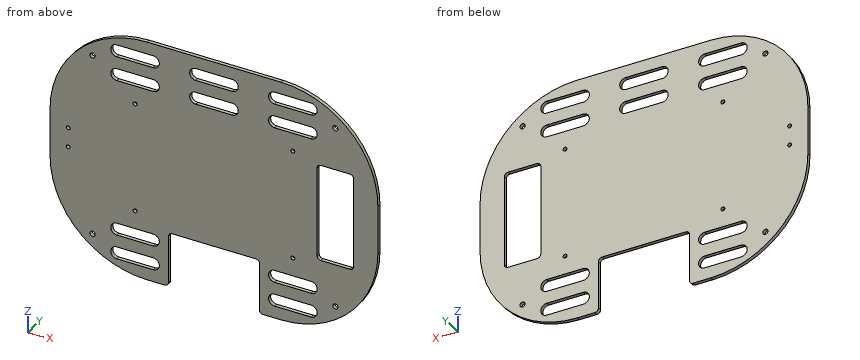
from build123d import *

# Parameters (mm, degrees)
SKETCH_1_W          = 270
SKETCH_1_H          = 200
EXTRUDE_1_DEPTH     = 3
SKETCH_2_R          = 2.15
CUT_EXTRUDE_1_DEPTH = 3
SKETCH_3_R          = 1.6
CUT_EXTRUDE_2_DEPTH = 3
SKETCH_4_W          = 75
SKETCH_4_H          = 45
CUT_EXTRUDE_3_DEPTH = 3
SKETCH_5_R          = 1.6
CUT_EXTRUDE_4_DEPTH = 3
SKETCH_6_W          = 30
SKETCH_6_H          = 80
CUT_EXTRUDE_5_DEPTH = 3
CUT_EXTRUDE_6_DEPTH = 3
FILLET_1_R          = 3


with BuildPart() as part:
    # 草图1 → 凸台-拉伸1 (new body)
    with BuildSketch(Plane(origin=(0, 0, 0), x_dir=(1, 0, 0), z_dir=(0, 1, 0))):
        Rectangle(SKETCH_1_W, SKETCH_1_H)
    extrude(amount=EXTRUDE_1_DEPTH)

    # 草图2 → 切除-拉伸1 (cut)
    with BuildSketch(Plane(origin=(0, 3, 0), x_dir=(1, 0, 0), z_dir=(0, 1, 0))):
        with Locations(Location((-100, 75, 0), (0, 0, 270))):
            Circle(SKETCH_2_R)
        with Locations(Location((100, 75, 0), (0, 0, 270))):
            Circle(SKETCH_2_R)
        with Locations(Location((100, -75, 0), (0, 0, 270))):
            Circle(SKETCH_2_R)
        with Locations(Location((-100, -75, 0), (0, 0, 270))):
            Circle(SKETCH_2_R)
    extrude(amount=-CUT_EXTRUDE_1_DEPTH, mode=Mode.SUBTRACT)

    # 草图3 → 切除-拉伸2 (cut)
    with BuildSketch(Plane(origin=(0, 3, 0), x_dir=(1, 0, 0), z_dir=(0, 1, 0))):
        with Locations(Location((-120, 8, 0), (0, 0, 270))):
            Circle(SKETCH_3_R)
        with Locations(Location((-120, -8, 0), (0, 0, 270))):
            Circle(SKETCH_3_R)
    extrude(amount=-CUT_EXTRUDE_2_DEPTH, mode=Mode.SUBTRACT)

    # 草图4 → 切除-拉伸3 (cut)
    with BuildSketch(Plane(origin=(0, 3, 0), x_dir=(1, 0, 0), z_dir=(0, 1, 0))):
        with BuildLine():
            Line((-80, -80), (-50, -80))
            ThreePointArc((-50, -80), (-45, -85), (-50, -90))
            Line((-50, -90), (-80, -90))
            ThreePointArc((-80, -90), (-85, -85), (-80, -80))
        make_face()
        with BuildLine():
            Line((-15, -80), (15, -80))
            ThreePointArc((15, -80), (20, -85), (15, -90))
            Line((15, -90), (-15, -90))
            ThreePointArc((-15, -90), (-20, -85), (-15, -80))
        make_face()
        with BuildLine():
            Line((50, -80), (80, -80))
            ThreePointArc((80, -80), (85, -85), (80, -90))
            Line((80, -90), (50, -90))
            ThreePointArc((50, -90), (45, -85), (50, -80))
        make_face()
        with BuildLine():
            Line((-15, -60), (15, -60))
            ThreePointArc((15, -60), (20, -65), (15, -70))
            Line((15, -70), (-15, -70))
            ThreePointArc((-15, -70), (-20, -65), (-15, -60))
        make_face()
        with BuildLine():
            Line((50, -60), (80, -60))
            ThreePointArc((80, -60), (85, -65), (80, -70))
            Line((80, -70), (50, -70))
            ThreePointArc((50, -70), (45, -65), (50, -60))
        make_face()
        with BuildLine():
            Line((-80, -60), (-50, -60))
            ThreePointArc((-50, -60), (-45, -65), (-50, -70))
            Line((-50, -70), (-80, -70))
            ThreePointArc((-80, -70), (-85, -65), (-80, -60))
        make_face()
        with BuildLine():
            Line((-80, 80), (-50, 80))
            ThreePointArc((-50, 80), (-45, 85), (-50, 90))
            Line((-50, 90), (-80, 90))
            ThreePointArc((-80, 90), (-85, 85), (-80, 80))
        make_face()
        with BuildLine():
            Line((50, 80), (80, 80))
            ThreePointArc((80, 80), (85, 85), (80, 90))
            Line((80, 90), (50, 90))
            ThreePointArc((50, 90), (45, 85), (50, 80))
        make_face()
        with BuildLine():
            Line((50, 60), (80, 60))
            ThreePointArc((80, 60), (85, 65), (80, 70))
            Line((80, 70), (50, 70))
            ThreePointArc((50, 70), (45, 65), (50, 60))
        make_face()
        with BuildLine():
            Line((-80, 60), (-50, 60))
            ThreePointArc((-50, 60), (-45, 65), (-50, 70))
            Line((-50, 70), (-80, 70))
            ThreePointArc((-80, 70), (-85, 65), (-80, 60))
        make_face()
        with Locations((0, 77.5)):
            Rectangle(SKETCH_4_W, SKETCH_4_H)
    extrude(amount=-CUT_EXTRUDE_3_DEPTH, mode=Mode.SUBTRACT)

    # 草图5 → 切除-拉伸4 (cut)
    with BuildSketch(Plane(origin=(0, 3, 0), x_dir=(1, 0, 0), z_dir=(0, 1, 0))):
        with Locations(Location((-65, -45, 0), (0, 0, 270))):
            Circle(SKETCH_5_R)
        with Locations(Location((-65, 45, 0), (0, 0, 270))):
            Circle(SKETCH_5_R)
        with Locations(Location((65, 45, 0), (0, 0, 270))):
            Circle(SKETCH_5_R)
        with Locations(Location((65, -45, 0), (0, 0, 270))):
            Circle(SKETCH_5_R)
    extrude(amount=-CUT_EXTRUDE_4_DEPTH, mode=Mode.SUBTRACT)

    # 草图6 → 切除-拉伸5 (cut)
    with BuildSketch(Plane(origin=(0, 3, 0), x_dir=(1, 0, 0), z_dir=(0, 1, 0))):
        with Locations((100, 0)):
            Rectangle(SKETCH_6_W, SKETCH_6_H)
    extrude(amount=-CUT_EXTRUDE_5_DEPTH, mode=Mode.SUBTRACT)

    # 草图7 → 切除-拉伸6 (cut)
    with BuildSketch(Plane(origin=(0, 3, 0), x_dir=(1, 0, 0), z_dir=(0, 1, 0))):
        with BuildLine():
            Line((-55, 100), (-135, 100))
            Line((-135, 100), (-135, 20))
            ThreePointArc((-135, 20), (-111.568542495, 76.568542495), (-55, 100))
        make_face()
        with BuildLine():
            Line((-135, -100), (-135, -20))
            ThreePointArc((-135, -20), (-111.568542495, -76.568542495), (-55, -100))
            Line((-55, -100), (-135, -100))
        make_face()
        with BuildLine():
            Line((55, -100), (135, -100))
            Line((135, -100), (135, -20))
            ThreePointArc((135, -20), (111.568542495, -76.568542495), (55, -100))
        make_face()
        with BuildLine():
            Line((135, 100), (135, 20))
            ThreePointArc((135, 20), (111.568542495, 76.568542495), (55, 100))
            Line((55, 100), (135, 100))
        make_face()
    extrude(amount=-CUT_EXTRUDE_6_DEPTH, mode=Mode.SUBTRACT)

    # 圆角1
    fillet_1_edges = [part.edges().sort_by_distance(p)[0] for p in [
        (-37.5, 1.5, -55),
        (-37.5, 1.5, -100),
        (37.5, 1.5, -100),
        (37.5, 1.5, -55),
        (115, 1.5, -40),
        (115, 1.5, 40),
        (85, 1.5, 40),
        (85, 1.5, -40),
    ]]
    fillet(fillet_1_edges, radius=FILLET_1_R)


solid = part.part
Build history of the part. All positions in model axes, mm. Give positions to 0.01 mm unless a question says otherwise; leave off trailing zeros. Loops run counter-clockwise (first coordinate to the right, second up) from the corner with the lowest first, then second, coordinate; pieces in that order, holes last. Notation, with made-up numbers: (-19, -14.5) - (35, -14.5) arc R30 cw to (35, 10.5) - close; hole circle Ø6 at (77, 87). An arc over 180 degrees is marked (long way). Write item = value, one per line. Start each with the question number.
1) Band-saw the part on A-A on x = 73.5. Give the cut face in (y, z), plus the area to 3 significant figures.
2) Band-saw the part on B-B on z = 85. Give the cut face in (x, y).
3) Drop flat-ended pins along their axis: pin 1 Ø1.5 at (x, y) = (62, 1) entering from -Z; pin 2 Ø0.9 at (y, z) = (1, -75) entering from -X; pin 3 Ø0.9 at (x, y) = (-64, 2) entering from -Z. Give the stop position or say it passes through.
4) Probe probe 1 along Z at (x, y) = (55, 0.75); probe 2 along Z at (x, y) = (-120, 2.3); probe 3 along Z at (x, y) = (-9.5, 0.5). List the from-to ranges inside material, lowest first. Write a range as from..to.
5) Band-saw the part on C-C on y = 0.6. Count the separate pieces of the cut face and the enclosed holes in it, plus the area to 3 significant figures.
Final values:
q1.outline = (0, -97.83) - (3, -97.83) - (3, -90) - (0, -90) - close; (0, -80) - (3, -80) - (3, -70) - (0, -70) - close; (0, -60) - (3, -60) - (3, 60) - (0, 60) - close; (0, 70) - (3, 70) - (3, 80) - (0, 80) - close; (0, 90) - (3, 90) - (3, 97.83) - (0, 97.83) - close
q1.area = 467 mm²
q2.outline = (-101.64, 0) - (-85, 0) - (-85, 3) - (-101.64, 3) - close; (-45, 0) - (-20, 0) - (-20, 3) - (-45, 3) - close; (20, 0) - (45, 0) - (45, 3) - (20, 3) - close; (85, 0) - (101.64, 0) - (101.64, 3) - (85, 3) - close
q3.pin_1 = -99.76
q3.pin_2 = -113.52
q3.pin_3 = -99.54
q4.probe_1 = -100..-90, -80..-70, -60..60, 70..80, 90..100
q4.probe_2 = -66.64..-9.6, -6.4..6.4, 9.6..66.64
q4.probe_3 = -55..60, 70..80, 90..100
q5.separate_pieces = 1
q5.enclosed_holes = 21
q5.area = 38,800 mm²
